from build123d import *

# Parameters (mm, degrees)
BOSS_EXTRUDE1_DEPTH = 25.4
SKETCH2_R           = 1.27
CUT_EXTRUDE1_DEPTH  = 25.4


with BuildPart() as part:
    # Sketch1 → Boss-Extrude1 (new body)
    with BuildSketch(Plane(origin=(0, 0, 0), x_dir=(0, 0, -1), z_dir=(1, 0, 0))):
        Polygon((0, 0), (0, 12.7), (-3.175, 12.7), (-3.175, -3.175), (10.668, -3.175), (10.668, 0), align=None)
    extrude(amount=BOSS_EXTRUDE1_DEPTH)

    # Sketch2 → Cut-Extrude1 (cut)
    with BuildSketch(Plane.XY.offset(3.175)):
        with Locations((6.35, 3.175)):
            Circle(SKETCH2_R)
        with Locations((19.05, 3.175)):
            Circle(SKETCH2_R)
    extrude(amount=-CUT_EXTRUDE1_DEPTH, mode=Mode.SUBTRACT)


solid = part.part
Here's how the part is built. I have some questions about the finished solid (model axes, mm). A direction names the side the tool comes from. Round coordinates to 2 decimals unless told otherwise and drop trailing zeros. Loops run counter-clockwise (first coordinate to the right, second up) from the corner with the lowest first, then second, coordinate; pieces in that order, holes last. Notation, with made-up numbers: (35.25, 88.5) - (80.25, 88.5) arc R20 ccw to (80.25, 115.5) - close; hole circle Ø1 at (24, -30.75). An arc over 180 degrees is marked (long way). One line per question, with ' | ' between items. Start each with the question number.
Q1. I want a section at C-C (y = 2.5). Write out the boundary of the cut face in (x, z) (3 decimals), then the cut area to 3 significant figures.
Q2. I want a section at B-B (z = 0.5). Write out the boundary of the cut face in (x, y) (3 decimals), then the cut area to 3 significant figures.
Q3. Will these pins go through, and if not, where does the flat tip stop? pin 1 (1.5 mm diameter, centred on x = 6.35, y = 3.175, fed in from +Z); pin 2 (8 mm diameter, centred on x = 6, z = -7, fed in from +Y); pin 3 (3 mm diameter, centred on x = 20, y = 10, fed in from -Z).
Q4. We'd pull the mould along X, two halves only. Please class faces 1 (the cylindrical face through (6.185, 4.434, 1.61)), 2 (the flat face through (25.4, 1, 1)), 3 (the cylindrical face through (17.78, 3.23, 1.61)), 4 (the flat face through (13, 5, 3.175)): +X half, -X half, draft (parallel to the pull), parting line (faces both ways), or undercut.
Q5. For faces 5 (the flat face through (13, -3.175, -4)), 6 (the flat face through (13, 6, 0)), which set-ups out of +Z, -Z, +X, -X, +Y, -Y let a thin tool reach every point of the face, with its end or its side?
Q6. Please list where these lines run through material, in increasing order: line 1 (Y direction, x = 6.35, z = 2.55) (3 decimals); line 2 (Z direction, x = 13.75, y = 10.75) (3 decimals); line 3 (Y direction, x = 10.5, z = -7) (3 decimals). Write a range as [from, to].
Q7. I want a section at A-A (x = 19.05). Write out the boundary of the cut face in (y, z) (3 decimals), then the cut area to 3 significant figures.
Q8. I want a section at D-D (x = 9). Write out the boundary of the cut face in (y, z) (3 decimals).
Response values:
1) outline: (0, 0) - (5.274, 0) - (5.274, 3.175) - (0, 3.175) - close; (7.426, 0) - (17.974, 0) - (17.974, 3.175) - (7.426, 3.175) - close; (20.126, 0) - (25.4, 0) - (25.4, 3.175) - (20.126, 3.175) - close | area: 67.0 mm²
2) outline: (0, -3.175) - (25.4, -3.175) - (25.4, 12.7) - (0, 12.7) - close; hole circle Ø2.54 at (6.35, 3.175); hole circle Ø2.54 at (19.05, 3.175) | area: 393 mm²
3) pin 1: passes through | pin 2: stops at y = 0 | pin 3: stops at z = 0
4) face 1: undercut | face 2: +X half | face 3: undercut | face 4: draft
5) face 5: +Z, -Z, +X, -X, -Y | face 6: -Z, +X, -X, +Y
6) line 1: y = [-3.175, 1.905], [4.445, 12.7] | line 2: z = [0, 3.175] | line 3: y = [-3.175, 0]
7) outline: (-3.175, -10.668) - (0, -10.668) - (0, 0) - (1.905, 0) - (1.905, 3.175) - (-3.175, 3.175) - close; (4.445, 0) - (12.7, 0) - (12.7, 3.175) - (4.445, 3.175) - close | area: 76.2 mm²
8) outline: (-3.175, -10.668) - (0, -10.668) - (0, 0) - (12.7, 0) - (12.7, 3.175) - (-3.175, 3.175) - close
